Verification items for the finished model (mm, model axes). Give positions to 0.01 mm unless a question says otherwise; leave off trailing zeros. Loops run counter-clockwise (first coordinate to the right, second up) from the corner with the lowest first, then second, coordinate; pieces in that order, holes last. Notation, with made-up numbers: (-34.5, 64.25) -> (7.5, 64.25) arc R21 cw to (7.5, 70.25) -> close; hole circle Ø2 at (-5, -14.5). An arc over 180 degrees is marked (long way). Answer in a Markdown table with one row per item. Add a question column.
Q1. Material ranges on probe 1 along X at (y, z) = (152.5, -0.7); probe 2 along X at (y, z) = (164.5, -3.2); probe 3 along Y at (x, z) = (-65.5, -3.25), recorded low to high.
Q2. Section check B-B on x = -82.5. Enter the section's corners in (y, z), and give its area (3 significant figures).
Q3. Section check D-D on x = -5.5. Enter the section's corners in (y, z), and give its area (3 significant figures).
Q4. Section check C-C on z = -2.55. Give the number of separate pieces and of enclosed holes in the cut face, and give its area (3 significant figures).
Q5. Section check A-A on y = 75. Enter the section's corners in (x, z).
Q6. Gauge pin test, flat ends, axial feed: P1, Ø1.5, axis at x = -145.5, z = -1.5, coming from the +Y side; P2, Ø2.5, axis at y = 172, z = -3.5, coming from the +X side; P3, Ø3, axis at y = 126.5, z = -1, coming from the +X side. Record the tip position at first contact, or that the pin passes through.
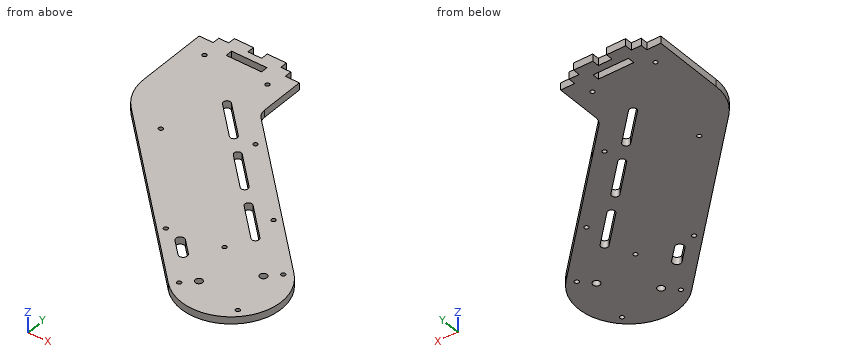
```python
from build123d import *

# Parameters (mm, degrees)
SKETCH1_R           = 1.475
SKETCH1_R_2         = 2.5
SKETCH1_W           = 24.7
SKETCH1_H           = 4.85
BOSS_EXTRUDE1_DEPTH = 5


with BuildPart() as part:
    # Sketch1 → Boss-Extrude1 (new body)
    with BuildSketch(Plane.XY):
        with BuildLine():
            Line((-139.300035894, 89.802561211), (-24.748737342, -24.748737342))
            ThreePointArc((-24.748737342, -24.748737342), (24.748737342, -24.748737342), (24.748737342, 24.748737342))
            Line((24.748737342, 24.748737342), (-54.672802234, 104.170276917))
            Line((-54.672802234, 104.170276917), (-76.622366364, 126.119841047))
            ThreePointArc((-76.622366364, 126.119841047), (-78.790093877, 129.364074535), (-79.551298552, 133.190908859))
            Line((-79.551298552, 133.190908859), (-79.551298552, 164.551298552))
            Line((-79.551298552, 164.551298552), (-89.351298552, 164.551298552))
            Line((-89.351298552, 164.551298552), (-89.351298552, 169.551298552))
            Line((-89.351298552, 169.551298552), (-96.351298552, 169.551298552))
            Line((-96.351298552, 169.551298552), (-96.351298552, 174.551298552))
            Line((-96.351298552, 174.551298552), (-109.751298552, 174.551298552))
            Line((-109.751298552, 174.551298552), (-109.751298552, 169.551298552))
            Line((-109.751298552, 169.551298552), (-119.351298552, 169.551298552))
            Line((-119.351298552, 169.551298552), (-119.351298552, 174.551298552))
            Line((-119.351298552, 174.551298552), (-132.751298552, 174.551298552))
            Line((-132.751298552, 174.551298552), (-132.751298552, 169.551298552))
            Line((-132.751298552, 169.551298552), (-139.751298552, 169.551298552))
            Line((-139.751298552, 169.551298552), (-139.751298552, 164.551298552))
            Line((-139.751298552, 164.551298552), (-149.551298552, 164.551298552))
            Line((-149.551298552, 164.551298552), (-149.551298552, 114.551298552))
            ThreePointArc((-149.551298552, 114.551298552), (-146.88708219, 101.157378419), (-139.300035894, 89.802561211))
        make_face()
        with Locations((-20.506096654, -20.506096654)):
            Circle(SKETCH1_R, mode=Mode.SUBTRACT)
        with Locations((-12.727922061, -12.727922061)):
            Circle(SKETCH1_R_2, mode=Mode.SUBTRACT)
        with Locations((-56.568542495, 14.142135624)):
            Circle(SKETCH1_R, mode=Mode.SUBTRACT)
        with BuildLine():
            ThreePointArc((-45.891723759, 8.555498392), (-45.891723759, 12.670859859), (-41.776362292, 12.670859859))
            Line((-41.776362292, 12.670859859), (-32.583974137, 3.478471703))
            ThreePointArc((-32.583974137, 3.478471703), (-32.583974137, -0.636889763), (-36.699335604, -0.636889763))
            Line((-36.699335604, -0.636889763), (-45.891723759, 8.555498392))
        make_face(mode=Mode.SUBTRACT)
        with Locations((20.506096654, -20.506096654)):
            Circle(SKETCH1_R, mode=Mode.SUBTRACT)
        with Locations((12.727922061, 12.727922061)):
            Circle(SKETCH1_R_2, mode=Mode.SUBTRACT)
        with Locations((-20.506096654, 20.506096654)):
            Circle(SKETCH1_R, mode=Mode.SUBTRACT)
        with BuildLine():
            ThreePointArc((-35.001785669, 56.922095886), (-35.001785669, 60.457629791), (-31.466251763, 60.457629791))
            Line((-31.466251763, 60.457629791), (-10.253048327, 39.244426356))
            ThreePointArc((-10.253048327, 39.244426356), (-10.253048327, 35.70889245), (-13.788582233, 35.70889245))
            Line((-13.788582233, 35.70889245), (-35.001785669, 56.922095886))
        make_face(mode=Mode.SUBTRACT)
        with Locations((-14.142135624, 56.568542495)):
            Circle(SKETCH1_R, mode=Mode.SUBTRACT)
        with Locations((20.506096654, 20.506096654)):
            Circle(SKETCH1_R, mode=Mode.SUBTRACT)
        with Locations((-114.551298552, 84.551298552)):
            Circle(SKETCH1_R, mode=Mode.SUBTRACT)
        with BuildLine():
            ThreePointArc((-101.4698231, 123.390133317), (-101.4698231, 126.925667223), (-97.934289194, 126.925667223))
            Line((-97.934289194, 126.925667223), (-76.721085759, 105.712463787))
            ThreePointArc((-76.721085759, 105.712463787), (-76.721085759, 102.176929881), (-80.256619665, 102.176929881))
            Line((-80.256619665, 102.176929881), (-101.4698231, 123.390133317))
        make_face(mode=Mode.SUBTRACT)
        with Locations((-64.396887007, 105.308740477)):
            Circle(SKETCH1_R, mode=Mode.SUBTRACT)
        with Locations((-136.551298552, 152.551298552)):
            Circle(SKETCH1_R, mode=Mode.SUBTRACT)
        with Locations((-114.551298552, 162.126298552)):
            Rectangle(SKETCH1_W, SKETCH1_H, mode=Mode.SUBTRACT)
        with Locations((-92.551298552, 152.551298552)):
            Circle(SKETCH1_R, mode=Mode.SUBTRACT)
        with BuildLine():
            ThreePointArc((-68.235804384, 90.156114601), (-68.235804384, 93.691648507), (-64.700270479, 93.691648507))
            Line((-64.700270479, 93.691648507), (-43.487067043, 72.478445072))
            ThreePointArc((-43.487067043, 72.478445072), (-43.487067043, 68.942911166), (-47.022600949, 68.942911166))
            Line((-47.022600949, 68.942911166), (-68.235804384, 90.156114601))
        make_face(mode=Mode.SUBTRACT)
    extrude(amount=-BOSS_EXTRUDE1_DEPTH)


solid = part.part
```
Taken from the geometry:
| question | item | result |
|---|---|---|
| 1 | probe 1 | x = -149.55 to -138.03, -135.08 to -94.03, -91.08 to -79.55 |
| 1 | probe 2 | x = -149.55 to -126.9, -102.2 to -79.55 |
| 1 | probe 3 | y = 16 to 87.42, 94.23 to 104.33, 106.29 to 115 |
| 2 | outline | (33, -5) -> (104.42, -5) -> (104.42, 0) -> (33, 0) -> close; (111.49, -5) -> (164.55, -5) -> (164.55, 0) -> (111.49, 0) -> close |
| 2 | area | 622 mm² |
| 3 | outline | (-34.57, -5) -> (55, -5) -> (55, 0) -> (-34.57, 0) -> close |
| 3 | area | 448 mm² |
| 4 | separate pieces | 1 |
| 4 | enclosed holes | 17 |
| 4 | area | 16,300 mm² |
| 5 | outline | (-124.5, -5) -> (-53.08, -5) -> (-53.08, 0) -> (-124.5, 0) -> close; (-46.01, -5) -> (-25.5, -5) -> (-25.5, 0) -> (-46.01, 0) -> close |
| 6 | P1 | stops at y = 164.55 |
| 6 | P2 | stops at x = -96.35 |
| 6 | P3 | stops at x = -75.5 |
